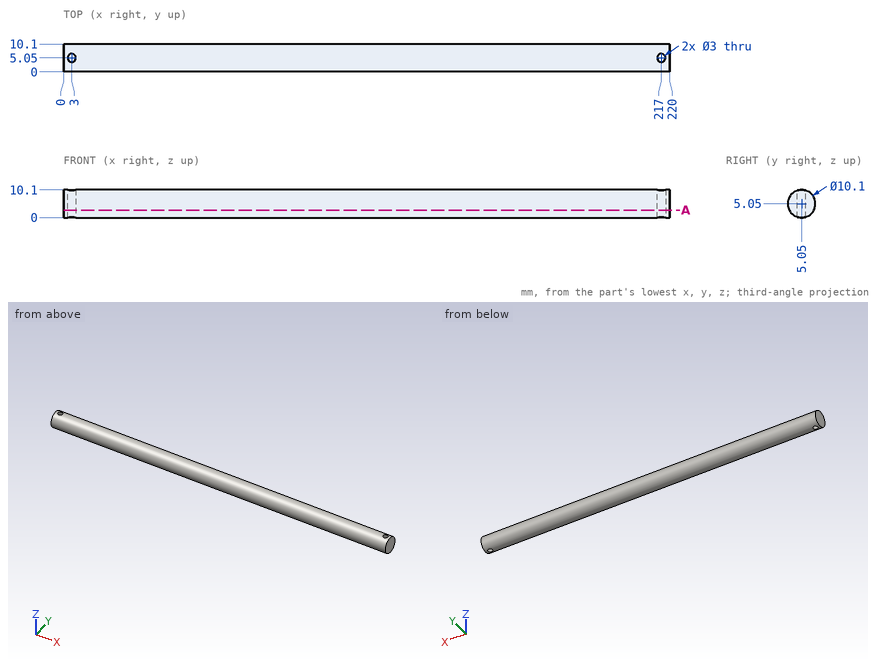
Answer from the drawing. Dimensions are ordinates in mm from the lowest x, y and z of the part. Give positions to 0.01 mm unless a question says otherwise; leave off trailing zeros. Loops run counter-clockwise (first coordinate to the right, second up) from the corner with the lowest first, then second, coordinate; pieces in that order, holes last. Notation, with made-up numbers: (67.5, 56) -> (115.5, 56) arc R11 ccw to (115.5, 75) -> close; hole circle Ø11 at (31, -17). An arc over 180 degrees is marked (long way). One line per question, with ' | ' between items. Start each with the question number.
1) Section A-A, the plane z = 2.75 is taken. Determine the outline of the cut face in (x, y).
2) Straight lines are drawn through the part: L1, parallel to X at y = 4.25, z = 1.5; L2, parallel to X at y = 6.25, z = 5.25; L3, parallel to Y at x = 184, z = 4.5. For each, find the intervals that lie inside material, in ascending order.
3) Each of these flat-tipped pins is pushed along its axis until it touches: pin 1 (5 mm diameter, centred on x = 194, z = 1, fed in from +Y); pin 2 (1.5 mm diameter, centred on x = 126.5, z = 4, fed in from +Y). Where does it stop, or does it pass through?
Resolved:
1) outline: (0, 0.55) -> (220, 0.55) -> (220, 9.55) -> (0, 9.55) -> close; hole circle Ø3 at (3, 5.05); hole circle Ø3 at (217, 5.05)
2) L1: 0 to 1.73, 4.27 to 215.73, 218.27 to 220 | L2: 0 to 2.1, 3.9 to 216.1, 217.9 to 220 | L3: 0.03 to 10.07
3) pin 1: y = 9.86 | pin 2: y = 10.09
